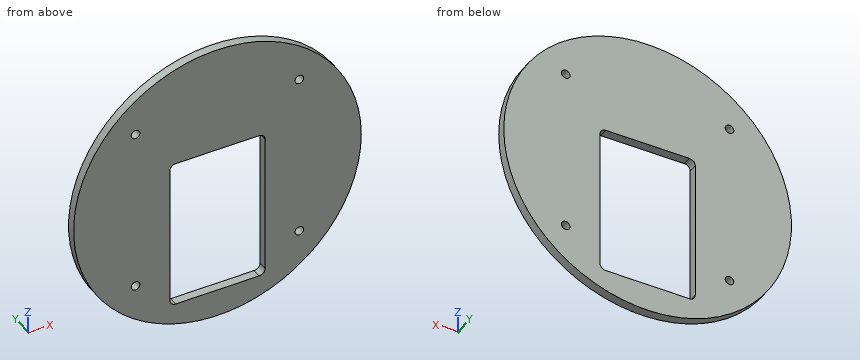
from build123d import *

# Parameters (mm, degrees)
F0_R     = 48.3
F1_DEPTH = 3
F2_R     = 1.25
F2_R_2   = 2.5
F3_DEPTH = 3.001
F4_R     = 1.45
F5_DEPTH = 3.001
F6_R     = 1
F7_DEPTH = 3.001
F8_W     = 32
F8_H     = 51
F9_DEPTH = 3.001
F10_R    = 2
F11_R    = 2
F12_R    = 2


with BuildPart() as f1:
    # F0 (on Front) → F1 (new body)
    with BuildSketch(Plane.XZ):
        Circle(F0_R)
    extrude(amount=F1_DEPTH)

    # F2 (on face) → F3 (cut, through all)
    with BuildSketch(Plane.XZ.offset(3)):
        with Locations((-8, 0)):
            Circle(F2_R)
        with Locations((8, 0)):
            Circle(F2_R)
        Circle(F2_R_2)
    extrude(amount=-F3_DEPTH, mode=Mode.SUBTRACT)

    # F4 (on face) → F5 (cut, through all)
    with BuildSketch(Plane.XZ.offset(3)):
        with Locations((-27.5, 27.5)):
            Circle(F4_R)
        with Locations((27.5, 27.5)):
            Circle(F4_R)
        with Locations((-27.5, -27.5)):
            Circle(F4_R)
        with Locations((27.5, -27.5)):
            Circle(F4_R)
    extrude(amount=-F5_DEPTH, mode=Mode.SUBTRACT)

    # F6 (on face) → F7 (cut, through all)
    with BuildSketch(Plane.XZ.offset(3)):
        with BuildLine():
            Line((-10.05, -33), (10.05, -33))
            Line((10.05, -33), (10.05, -5.589946))
            ThreePointArc((10.05, -5.589946), (0, -11.5), (-10.05, -5.589946))
            Line((-10.05, -5.589946), (-10.05, -33))
        make_face()
        with BuildLine():
            Line((10.05, 0), (10.05, -5.589946))
            ThreePointArc((10.05, -5.589946), (11.131599, -2.887473), (11.5, 0))
            ThreePointArc((11.5, 0), (-2.887473, 11.131599), (-10.05, -5.589946))
            Line((-10.05, -5.589946), (-10.05, 0))
            Line((-10.05, 0), (10.05, 0))
        make_face()
        with Locations((-13.5, -6.5)):
            Circle(F6_R)
        with Locations((-13.5, -14.5)):
            Circle(F6_R)
        with Locations((-13.5, -22.5)):
            Circle(F6_R)
        with Locations((-13.5, -30.5)):
            Circle(F6_R)
        with Locations((13.5, -6.5)):
            Circle(F6_R)
        with Locations((13.5, -14.5)):
            Circle(F6_R)
        with Locations((13.5, -22.5)):
            Circle(F6_R)
        with Locations((13.5, -30.5)):
            Circle(F6_R)
        with Locations((-8, -36)):
            Circle(F6_R)
        with Locations((8, -36)):
            Circle(F6_R)
    extrude(amount=-F7_DEPTH, mode=Mode.SUBTRACT)

    # F8 (on face) → F9 (cut, through all)
    with BuildSketch(Plane.XZ.offset(3)):
        with Locations((0, -13.5)):
            Rectangle(F8_W, F8_H)
    extrude(amount=-F9_DEPTH, mode=Mode.SUBTRACT)

    # F10
    f10_edges = [f1.edges().sort_by_distance(p)[0] for p in [
        (-16, -1.5, 12),
    ]]
    fillet(f10_edges, radius=F10_R)

    # F11
    f11_edges = [f1.edges().sort_by_distance(p)[0] for p in [
        (16, -1.5, 12),
    ]]
    fillet(f11_edges, radius=F11_R)

    # F12
    f12_edges = [f1.edges().sort_by_distance(p)[0] for p in [
        (16, -1.5, -39),
        (-16, -1.5, -39),
    ]]
    fillet(f12_edges, radius=F12_R)


solid = f1.part
Geometry check sheet. Reference: the model listing, model coordinates, mm. Round coordinates to 2 decimals unless told otherwise and drop trailing zeros. Write each loop counter-clockwise with the first axis right and the second up, starting at its lowest first coordinate (ties: lowest second). Pieces come first, ordered by that corner, then holes.
Item 1: Material ranges on line 1 along Z through (x, y) = (-27.5, -1.35); line 2 along X through (y, z) = (-0.3, -1); line 3 along X through (y, z) = (-1.65, -34.5), recorded low to high.
Determined:
line 1: z = -39.71 to -28.95, -26.05 to 26.05, 28.95 to 39.71
line 2: x = -48.29 to -16, 16 to 48.29
line 3: x = -33.8 to -16, 16 to 33.8
Item 2: Section check A-A (y = -1.1). Record the boundary of the cut face in (x, z).
Determined:
outline: circle Ø96.6 at (0, 0); hole circle Ø2.9 at (-27.5, -27.5); hole circle Ø2.9 at (-27.5, 27.5); hole (-16, -37) arc R2 ccw to (-14, -39) - (14, -39) arc R2 ccw to (16, -37) - (16, 10) arc R2 ccw to (14, 12) - (-14, 12) arc R2 ccw to (-16, 10) - close; hole circle Ø2.9 at (27.5, -27.5); hole circle Ø2.9 at (27.5, 27.5)
Item 3: Section check D-D (x = 27.5). Record the boundary of the cut face in (y, z), plus the area to 3 significant figures.
Determined:
outline: (-3, -39.71) - (0, -39.71) - (0, -28.95) - (-3, -28.95) - close; (-3, -26.05) - (0, -26.05) - (0, 26.05) - (-3, 26.05) - close; (-3, 28.95) - (0, 28.95) - (0, 39.71) - (-3, 39.71) - close
area: 221 mm2
Item 4: Section check C-C (z = -11.5). Record the boundary of the cut face in (x, y), plus the area to 3 significant figures.
Determined:
outline: (-46.91, -3) - (-16, -3) - (-16, 0) - (-46.91, 0) - close; (16, -3) - (46.91, -3) - (46.91, 0) - (16, 0) - close
area: 185 mm2
Item 5: Section check B-B (x = -2.5). Record the boundary of the cut face in (y, z), plus the area to 3 significant figures.
Determined:
outline: (-3, -48.24) - (0, -48.24) - (0, -39) - (-3, -39) - close; (-3, 12) - (0, 12) - (0, 48.24) - (-3, 48.24) - close
area: 136 mm2
Item 6: Go/stop test with flat-tipped pins: pin 1 Ø2.5 at (x, z) = (27.5, -27.5) entering from +Y; pin 2 Ø0.9 at (y, z) = (-1, -5.5) entering from +X; pin 3 Ø0.9 at (y, z) = (-2, -18.5) entering from -X. Record where each tip stops, or that it passes through.
Determined:
pin 1: passes through
pin 2: stops at x = 48.04
pin 3: stops at x = -44.8
